Can you work these out from the drawing? Everything is in mm from the part's minimum corner. A direction names the side the tool comes from. Coordinates: 2 decimals unless noted, no trailing zeros. Loops run counter-clockwise (first coordinate to the right, second up) from the corner with the lowest first, then second, coordinate; pieces in that order, holes last.
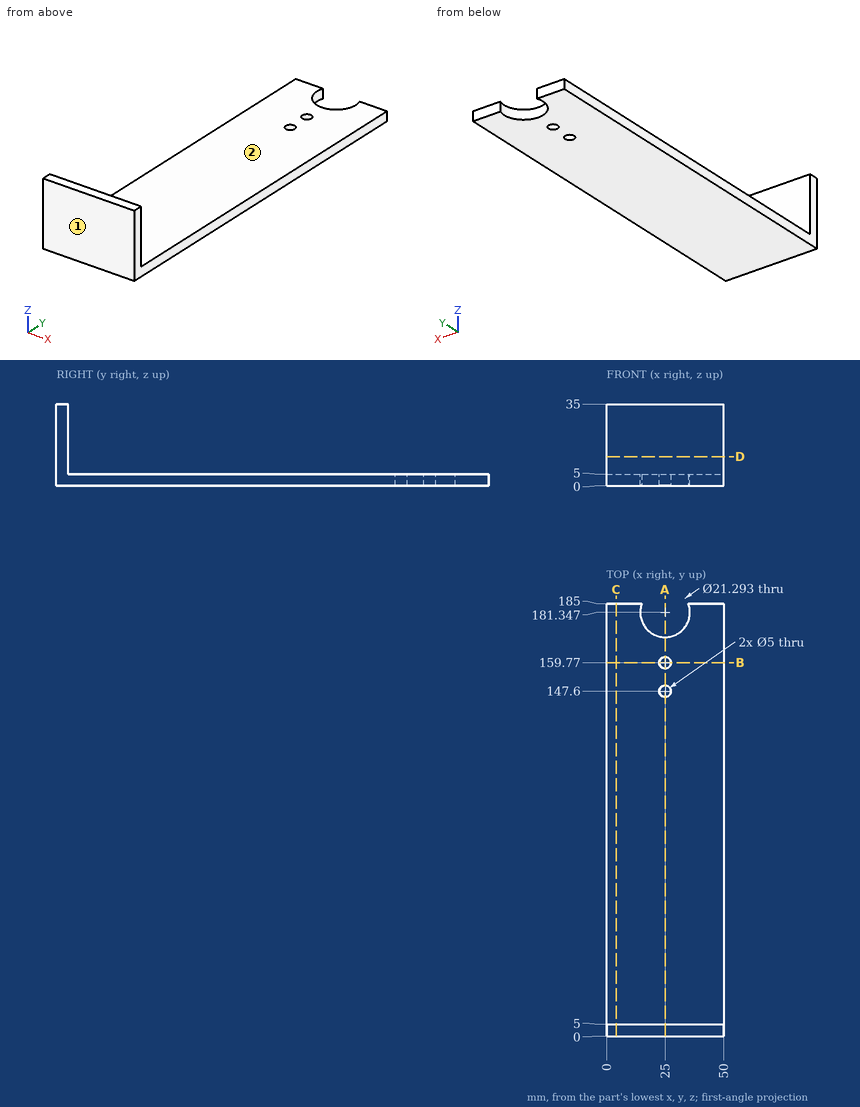
Item 1: Suppose I cut it at B-B, the plane y = 159.77. Please give me the cut outline in (x, z).
Results are:
outline: (0, 0) - (22.5, 0) - (22.5, 5) - (0, 5) - close; (27.5, 0) - (50, 0) - (50, 5) - (27.5, 5) - close
Item 2: Suppose I cut it at C-C, the plane x = 4. Please give me the cut outline in (y, z).
Results are:
outline: (0, 0) - (185, 0) - (185, 5) - (5, 5) - (5, 35) - (0, 35) - close
Item 3: Suppose I cut it at D-D, the plane z = 12.5. Please give me the cut outline in (x, y), plus the area to 3 significant figures.
Results are:
outline: (0, 0) - (50, 0) - (50, 5) - (0, 5) - close
area: 250 mm2
Item 4: On a 3-axis mill with a long thin cutter (end or side, diameter ignored), from which of +Z, -Z, +X, -X, +Y, -Y can I reach the whole of each face in a straight line? I mean the marked faces 1 and 2. Say none if no direction works.
Results are:
face 1: +Z, -Z, +X, -X, -Y
face 2: +Z, +X, -X, +Y
Item 5: I'm going to push flat-ended pins straight in: P1, Ø2, axis at x = 25, z = 26, coming from the +Y side; P2, Ø5, axis at x = 7, y = 94.5, coming from the +Z side. Where does each tip first touch, or does it pass through?
Results are:
P1: stops at y = 5
P2: stops at z = 5
Item 6: Suppose I cut it at A-A, the plane x = 25. Please give me the cut outline in (y, z).
Results are:
outline: (0, 0) - (145.1, 0) - (145.1, 5) - (5, 5) - (5, 35) - (0, 35) - close; (150.1, 0) - (157.27, 0) - (157.27, 5) - (150.1, 5) - close; (162.27, 0) - (170.7, 0) - (170.7, 5) - (162.27, 5) - close
Item 7: I need wall thicknesses on line 1 along Y through (x, z) = (25, 2.65); line 2 along X through (y, z) = (147.6, 3.8); line 3 along Z through (x, y) = (8.5, 59). Which ranges of each line are inside material? Lowest first, please.
Results are:
line 1: y = 0 to 145.1, 150.1 to 157.27, 162.27 to 170.7
line 2: x = 0 to 22.5, 27.5 to 50
line 3: z = 0 to 5
